Verification items for the finished model (mm, model axes). A direction names the side the tool comes from. Give positions to 0.01 mm unless a question says otherwise; leave off trailing zeros. Write each loop counter-clockwise with the first axis right and the second up, starting at its lowest first coordinate (ties: lowest second). Pieces come first, ordered by that corner, then holes. Notation, with made-up numbers: (18.25, -39.5) -> (37.25, -39.5) arc R24 ccw to (37.25, -2.5) -> close; hole circle Ø8 at (7.25, 24.5). An arc over 180 degrees is marked (long way). Answer as CSV lines item,"result".
```python
from build123d import *

# Parameters (mm, degrees)
SKETCH_1_R      = 10
EXTRUDE_1_DEPTH = 90
SKETCH_2_W      = 35
SKETCH_2_H      = 20
EXTRUDE_2_DEPTH = 10
SKETCH_3_R      = 4
EXTRUDE_3_DEPTH = 5
SKETCH_5_W      = 35
SKETCH_5_H      = 35
EXTRUDE_4_DEPTH = 10


with BuildPart() as part:
    # 草图1 → 凸台-拉伸1 (new body)
    with BuildSketch(Plane(origin=(0, 0, 0), x_dir=(0, 0, -1), z_dir=(1, 0, 0))):
        with Locations(Location((0, 0, 0), (0, 0, 180))):
            Circle(SKETCH_1_R)
    extrude(amount=EXTRUDE_1_DEPTH)

    # 草图2 → 凸台-拉伸2 (add)
    with BuildSketch(Plane.XY):
        with Locations((72.5, 0)):
            Rectangle(SKETCH_2_W, SKETCH_2_H)
    extrude(amount=EXTRUDE_2_DEPTH)

    # 草图3 → 凸台-拉伸3 (add)
    with BuildSketch(Plane.XY.offset(10)):
        with Locations((81.45858647, 0)):
            Circle(SKETCH_3_R)
    extrude(amount=EXTRUDE_3_DEPTH)

    # 草图5 → 凸台-拉伸4 (add)
    with BuildSketch(Plane.ZY):
        Rectangle(SKETCH_5_W, SKETCH_5_H)
    extrude(amount=EXTRUDE_4_DEPTH)


solid = part.part
```
1) Tool access check on faces 1 (the flat face through (72, -10, 5)), 2 (the flat face through (55, 8, 8)), 3 (the cylindrical face through (77.462, 0.176, 12.465)), 4 (the flat face through (81, 0, 15)), 5 (the flat face through (55, -8, 8)). Record the directions out of +Z, -Z, +X, -X, +Y, -Y that give a thin tool (end or side, any length) a straight path to the whole face; none if there is none.
Reported:
face 1,"+Z, -Z, +X, -Y"
face 2,"+Z, +Y"
face 3,"+Z"
face 4,"+Z, +X, +Y, -Y"
face 5,"+Z, -Y"
2) Scan lines: line 1 along X through (y, z) = (-9.5, 4); line 2 along X through (y, z) = (-6, -15.5); line 3 along Z through (x, y) = (58, 3.5). Record each from-to range of solid material in increasing order.
Reported:
line 1,"-10 to 0, 55 to 90"
line 2,"-10 to 0"
line 3,"-9.37 to 10"
3) Section check C-C (x = 37). Record the boundary of the cut face in (y, z).
Reported:
outline,"circle Ø20 at (0, 0)"
4) Section check B-B (y = 13.5). Record the boundary of the cut face in (x, z).
Reported:
outline,"(-10, -17.5) -> (0, -17.5) -> (0, 17.5) -> (-10, 17.5) -> close"
5) Depth check by flat-ended pin: pin 1 (4 mm diameter, centred on x = 30.5, z = -3, fed in from +Y); pin 2 (12 mm diameter, centred on y = 6, z = -11.5, fed in from +X); pin 3 (3 mm diameter, centred on x = 69.5, z = 6.5, fed in from -Y); pin 4 (3 mm diameter, centred on x = 69.5, z = 2.5, fed in from +Y). Enter the tip coordinate at first touch or a pass-through.
Reported:
pin 1,"y = 9.95"
pin 2,"x = 90"
pin 3,"y = -10"
pin 4,"y = 10"
6) Section check A-A (z = 3). Record the boundary of the cut face in (x, y), and give its area (3 significant figures).
Reported:
outline,"(-10, -17.5) -> (0, -17.5) -> (0, -9.54) -> (55, -9.54) -> (55, -10) -> (90, -10) -> (90, 10) -> (55, 10) -> (55, 9.54) -> (0, 9.54) -> (0, 17.5) -> (-10, 17.5) -> close"
area,"2,100 mm²"
7) Section check D-D (z = -7). Record the boundary of the cut face in (x, y).
Reported:
outline,"(-10, -17.5) -> (0, -17.5) -> (0, -7.14) -> (90, -7.14) -> (90, 7.14) -> (0, 7.14) -> (0, 17.5) -> (-10, 17.5) -> close"
8) Draft check along X on faces 6 (the flat face through (-5, 17.5, 0)), 7 (the flat face through (90, 0, 0)), 8 (the cylindrical face through (34, 0, -10)), 9 (the flat face through (-10, 0, 0)). Enter one of: +X half, -X half, draft (parallel to the pull), parting line (faces both ways), or undercut.
Reported:
face 6,"draft"
face 7,"+X half"
face 8,"undercut"
face 9,"-X half"
